For this review, take the finished solid that the model builds, in its own axes (mm). A direction names the side the tool comes from. Round coordinates to 2 decimals unless told otherwise and drop trailing zeros. Write each loop counter-clockwise with the first axis right and the second up, starting at its lowest first coordinate (ties: lowest second). Pieces come first, ordered by that corner, then holes. Notation, with made-up numbers: (53.5, -4.5) -> (71.5, -4.5) arc R24 cw to (71.5, 25.5) -> close; hole circle Ø7 at (2, 49.25). An arc over 180 degrees is marked (long way). Write each question's results on one line, items separated by ' | '. Start each with the question number.
Item 1: Add section A-A (z = 7.5). State the section outline as (x, y) points, plus the area to 3 significant figures.
Item 2: Tool access review of faces 4 (the flat face through (19, 4.5, 7)), 5 (the cylindrical face through (13.5, 6.02, 3.93)): name each direction out of +Z, -Z, +X, -X, +Y, -Y from which nothing blocks a thin tool from reaching the whole face with its end or side.
Item 3: Add section B-B (y = 5.5). State the section outline as (x, z) points.
Item 4: Add section D-D (x = 28.5). State the section outline as (y, z) points.
Item 5: Clearance check with flat-ended pins moving along their axes: pin 1 (1 mm diameter, centred on x = 12.5, z = 10.5, fed in from -Y); pin 2 (4 mm diameter, centred on y = -3.5, z = 2, fed in from +X). State where each tip first meets the part, or that it passes through.
Item 6: To check wall thickness, follow line 1 along Z through (x, y) = (15, 6.35); line 2 along X through (y, z) = (6.9, 11); line 3 along Z through (x, y) = (28.5, 5.75). State the ranges of each line that lie inside material, in increasing order.
Item 7: Add section C-C (z = 4). State the section outline as (x, y) points, plus the area to 3 significant figures.
Item 8: The part is to be moulded in two halves that separate along Y. For faces 1 (the cylindrical face through (30.47, 6.02, 6.88)), 2 (the flat face through (0, -7.5, 7)), 3 (the cylindrical face through (0.02, -0.43, 13)), say which applies: +Y half, -Y half, draft (parallel to the pull), parting line (faces both ways), or undercut.
from build123d import *

# Parameters (mm, degrees)
CROQUIS1_W              = 3
CROQUIS1_H              = 12
CROQUIS1_H_2            = 3
CROQUIS1_W_2            = 47
SALIENTE_EXTRUIR1_DEPTH = 15
CROQUIS2_R              = 1.5
CORTAR_EXTRUIR1_DEPTH   = 30
CROQUIS4_R              = 2.063665481
CORTAR_EXTRUIR3_DEPTH   = 10
CROQUIS5_W              = 11.835753584
CROQUIS5_H              = 15
CORTAR_EXTRUIR4_DEPTH   = 30
CROQUIS6_R              = 1.5
CORTAR_EXTRUIR5_DEPTH   = 10


with BuildPart() as part:
    # Croquis1 → Saliente-Extruir1 (new body)
    with BuildSketch(Plane.XY):
        with Locations((0, -1.5)):
            Rectangle(CROQUIS1_W, CROQUIS1_H)
        with Locations((0, 6)):
            Rectangle(CROQUIS1_W, CROQUIS1_H_2)
        with Locations((25, 6)):
            Rectangle(CROQUIS1_W_2, CROQUIS1_H_2)
    extrude(amount=SALIENTE_EXTRUIR1_DEPTH)

    # Croquis2 → Cortar-Extruir1 (cut)
    with BuildSketch(Plane(origin=(1.5, 0, 0), x_dir=(0, 0, -1), z_dir=(1, 0, 0))):
        with Locations((-11.5, -0.5)):
            Circle(CROQUIS2_R)
        with Locations((-4, -0.5)):
            Circle(CROQUIS2_R)
    extrude(amount=-CORTAR_EXTRUIR1_DEPTH, mode=Mode.SUBTRACT)

    # Croquis4 → Cortar-Extruir3 (cut)
    with BuildSketch(Plane(origin=(0, 7.5, 0), x_dir=(1, 0, 0), z_dir=(0, 1, 0))):
        with Locations((28.5, -7.5)):
            Circle(CROQUIS4_R)
    extrude(amount=-CORTAR_EXTRUIR3_DEPTH, mode=Mode.SUBTRACT)

    # Croquis5 → Cortar-Extruir4 (cut)
    with BuildSketch(Plane(origin=(0, 7.5, 0), x_dir=(1, 0, 0), z_dir=(0, 1, 0))):
        with Locations((42.582123208, -7.5)):
            Rectangle(CROQUIS5_W, CROQUIS5_H)
    extrude(amount=-CORTAR_EXTRUIR4_DEPTH, mode=Mode.SUBTRACT)

    # Croquis6 → Cortar-Extruir5 (cut)
    with BuildSketch(Plane(origin=(0, 7.5, 0), x_dir=(1, 0, 0), z_dir=(0, 1, 0))):
        with Locations((15, -4)):
            Circle(CROQUIS6_R)
        with Locations((15, -11)):
            Circle(CROQUIS6_R)
    extrude(amount=-CORTAR_EXTRUIR5_DEPTH, mode=Mode.SUBTRACT)


solid = part.part
Responses:
1) outline: (-1.5, -7.5) -> (1.5, -7.5) -> (1.5, 4.5) -> (26.44, 4.5) -> (26.44, 7.5) -> (-1.5, 7.5) -> close; (30.56, 4.5) -> (36.66, 4.5) -> (36.66, 7.5) -> (30.56, 7.5) -> close | area: 138 mm^2
2) face 4: +Z, -Z, +X, -Y | face 5: +Y, -Y
3) outline: (-1.5, 0) -> (36.66, 0) -> (36.66, 15) -> (-1.5, 15) -> close; hole circle Ø3 at (15, 4); hole circle Ø3 at (15, 11); hole circle Ø4.13 at (28.5, 7.5)
4) outline: (4.5, 0) -> (7.5, 0) -> (7.5, 5.44) -> (4.5, 5.44) -> close; (4.5, 9.56) -> (7.5, 9.56) -> (7.5, 15) -> (4.5, 15) -> close
5) pin 1: stops at y = 4.5 | pin 2: stops at x = 1.5
6) line 1: z = 0 to 2.5, 5.5 to 9.5, 12.5 to 15 | line 2: x = -1.5 to 13.5, 16.5 to 36.66 | line 3: z = 0 to 5.44, 9.56 to 15
7) outline: (-1.5, -7.5) -> (1.5, -7.5) -> (1.5, -2) -> (-1.5, -2) -> close; (-1.5, 1) -> (1.5, 1) -> (1.5, 4.5) -> (13.5, 4.5) -> (13.5, 7.5) -> (-1.5, 7.5) -> close; (16.5, 4.5) -> (36.66, 4.5) -> (36.66, 7.5) -> (16.5, 7.5) -> close | area: 132 mm^2
8) face 1: draft | face 2: -Y half | face 3: undercut
